```python
from build123d import *

# Parameters (mm, degrees)
BOSS_EXTRUDE1_DEPTH = 3
CUT_EXTRUDE1_REACH  = 69.03
SKETCH2_W           = 5
SKETCH2_H           = 35
BOSS_EXTRUDE8_DEPTH = 3
MIRROR1_DEPTH       = 3
FILLET1_R           = 2
FILLET2_R           = 10
FILLET3_R           = 6
FILLET4_R           = 1


# Read off the part's stored shape, not the designer's step: Mirror1
with BuildPart() as part:
    # Sketch1 → Boss-Extrude1 (new body)
    with BuildSketch(Plane.XY):
        with BuildLine():
            Line((-1.51, 0), (0, 0))
            Line((0, 0), (0, 5))
            Line((0, 5), (-1.51, 5))
            Line((-1.51, 5), (-1.51, 7))
            ThreePointArc((-1.51, 7), (-26.381774629, 5.897879108), (-50, -1.976082663))
            ThreePointArc((-50, -1.976082663), (-51.828078002, -17.5), (-50, -33.023917337))
            ThreePointArc((-50, -33.023917337), (-26.381774629, -40.897879108), (-1.51, -42))
            Line((-1.51, -42), (-1.51, -40))
            Line((-1.51, -40), (0, -40))
            Line((0, -40), (0, -35))
            Line((0, -35), (-1.51, -35))
            Line((-1.51, -35), (-1.51, -33))
            Line((-1.51, -33), (-1.51, -2))
            Line((-1.51, -2), (-1.51, 0))
        make_face()
    extrude(amount=BOSS_EXTRUDE1_DEPTH)

    # Sketch2 → Cut-Extrude1 (cut, up to next)
    with BuildSketch(Plane.XY.offset(3), mode=Mode.PRIVATE) as cut_extrude1_sk1:
        with BuildLine():
            ThreePointArc((-45.638636542, -5.430742036), (-46.828078002, -17.5), (-45.638636542, -29.569257964))
            ThreePointArc((-45.638636542, -29.569257964), (-26.536011476, -35.777357536), (-6.51, -37.329661985))
            Line((-6.51, -37.329661985), (-6.51, 2.329661985))
            ThreePointArc((-6.51, 2.329661985), (-26.536011476, 0.777357536), (-45.638636542, -5.430742036))
        make_face()
    cut_extrude1_tool1 = extrude(cut_extrude1_sk1.sketch, amount=-CUT_EXTRUDE1_REACH, mode=Mode.PRIVATE) & part.part
    # Sketch2 → Cut-Extrude1 (cut, up to next)
    with BuildSketch(Plane.XY.offset(3), mode=Mode.PRIVATE) as cut_extrude1_sk2:
        with Locations((-4.01, -17.5)):
            Rectangle(SKETCH2_W, SKETCH2_H)
    cut_extrude1_tool2 = extrude(cut_extrude1_sk2.sketch, amount=-CUT_EXTRUDE1_REACH, mode=Mode.PRIVATE) & part.part
    add(cut_extrude1_tool1.solids().sort_by_distance((-24.946194, -17.5, 3))[0], mode=Mode.SUBTRACT)
    add(cut_extrude1_tool2.solids().sort_by_distance((-4.01, -17.5, 3))[0], mode=Mode.SUBTRACT)

    # Sketch3 → Boss-Extrude8 (add)
    with BuildSketch(Plane.XY.offset(3)):
        with BuildLine():
            ThreePointArc((-32.612027687, -34.338487741), (-31.049231117, -34.753813219), (-29.478816537, -35.139334187))
            ThreePointArc((-29.478816537, -35.139334187), (-16.456843028, -24.361316901), (0, -20.5))
            Line((0, -20.5), (0, -14.5))
            ThreePointArc((0, -14.5), (-16.456843028, -10.638683099), (-29.478816537, 0.139334187))
            ThreePointArc((-29.478816537, 0.139334187), (-31.049231117, -0.246186781), (-32.612027687, -0.661512259))
            ThreePointArc((-32.612027687, -0.661512259), (-22.163998061, -10.798005795), (-8.780487851, -16.524390234))
            ThreePointArc((-8.780487851, -16.524390234), (-8, -17.499999784), (-8.780487429, -18.475609671))
            ThreePointArc((-8.780487429, -18.475609671), (-22.163997881, -24.201994085), (-32.612027687, -34.338487741))
        make_face()
    extrude(amount=-BOSS_EXTRUDE8_DEPTH)

    # Mirror1 outline → Mirror1 (add)
    with BuildSketch(Plane.XY):
        with BuildLine():
            ThreePointArc((29.478816537, -35.139334187), (18.069073524, -37.017473377), (6.51, -37.329661985))
            Line((6.51, -37.329661985), (6.51, -35))
            Line((6.51, -35), (0, -35))
            Line((0, -35), (0, -40))
            Line((0, -40), (1.51, -40))
            Line((1.51, -40), (1.51, -42))
            ThreePointArc((1.51, -42), (26.381774629, -40.897879108), (50, -33.023917337))
            ThreePointArc((50, -33.023917337), (51.828078002, -17.5), (50, -1.976082663))
            ThreePointArc((50, -1.976082663), (26.381774629, 5.897879108), (1.51, 7))
            Line((1.51, 7), (1.51, 5))
            Line((1.51, 5), (0, 5))
            Line((0, 5), (0, 0))
            Line((0, 0), (6.51, 0))
            Line((6.51, 0), (6.51, 2.329661985))
            ThreePointArc((6.51, 2.329661985), (18.069073524, 2.017473377), (29.478816537, 0.139334187))
            ThreePointArc((29.478816537, 0.139334187), (16.456843029, -10.638683099), (0, -14.5))
            Line((0, -14.5), (0, -20.5))
            ThreePointArc((0, -20.5), (16.456843029, -24.361316901), (29.478816537, -35.139334187))
        make_face()
        with BuildLine():
            ThreePointArc((45.638636542, -29.569257964), (39.22278835, -32.220063478), (32.612027687, -34.338487741))
            ThreePointArc((32.612027687, -34.338487741), (22.163998041, -24.201994192), (8.780487805, -18.475609756))
            ThreePointArc((8.780487805, -18.475609756), (8, -17.5), (8.780487805, -16.524390244))
            ThreePointArc((8.780487805, -16.524390244), (22.163998041, -10.798005808), (32.612027687, -0.661512259))
            ThreePointArc((32.612027687, -0.661512259), (39.22278835, -2.779936522), (45.638636542, -5.430742036))
            ThreePointArc((45.638636542, -5.430742036), (46.828078002, -17.5), (45.638636542, -29.569257964))
        make_face(mode=Mode.SUBTRACT)
    extrude(amount=MIRROR1_DEPTH)

    # Fillet1
    fillet1_edges = [part.edges().sort_by_distance(p)[0] for p in [
        (6.51, -35, 1.5),
        (6.51, 0, 1.5),
        (-6.51, 0, 1.5),
        (-6.51, -35, 1.5),
    ]]
    fillet(fillet1_edges, radius=FILLET1_R)

    # Fillet2
    fillet2_edges = [part.edges().sort_by_distance(p)[0] for p in [
        (-6.51, 2.329661985, 1.5),
        (6.51, 2.329661985, 1.5),
        (6.51, -37.329661985, 1.5),
        (-6.51, -37.329661985, 1.5),
    ]]
    fillet(fillet2_edges, radius=FILLET2_R)

    # Fillet3
    fillet3_edges = [part.edges().sort_by_distance(p)[0] for p in [
        (45.638636542, -5.430742036, 1.5),
        (45.638636542, -29.569257964, 1.5),
        (32.612027687, -0.661512259, 1.5),
        (32.612027687, -34.338487741, 1.5),
        (-50, -33.023917337, 1.5),
        (-50, -1.976082663, 1.5),
        (-45.638636542, -29.569257964, 1.5),
        (-45.638636542, -5.430742036, 1.5),
        (-32.612027687, -0.661512259, 1.5),
        (-32.612027687, -34.338487741, 1.5),
        (50, -1.976082663, 1.5),
        (50, -33.023917337, 1.5),
    ]]
    fillet(fillet3_edges, radius=FILLET3_R)

    # Fillet4
    fillet4_edges = [part.edges().sort_by_distance(p)[0] for p in [
        (29.478816537, 0.139334187, 1.5),
        (29.478816537, -35.139334187, 1.5),
        (-29.478816537, -35.139334187, 1.5),
        (-29.478816537, 0.139334187, 1.5),
    ]]
    fillet(fillet4_edges, radius=FILLET4_R)


solid = part.part
```
The model under review builds one solid part; all positions refer to its coordinate system, in mm. A direction names the side the tool comes from. Round coordinates to 2 decimals unless told otherwise and drop trailing zeros. Loops run counter-clockwise (first coordinate to the right, second up) from the corner with the lowest first, then second, coordinate; pieces in that order, holes last. Notation, with made-up numbers: (82.5, -36.5) - (101.5, -36.5) arc R18 cw to (101.5, -29.5) - close; hole circle Ø5 at (10, 7). An arc over 180 degrees is marked (long way). Use a Markdown table: item, result. Add a question column.
Q1. Add section B-B (y = -23). State the section outline as (x, z) points.
Q2. Add section D-D (y = 4). State the section outline as (x, z) points, plus the area to 3 significant figures.
Q3. The part is to be moulded in two halves that separate along X. For faces 5 (the face through (0, -19, 0)), 6 (the face through (51.828, -17.676, 1.479)), 7 (the face through (1.51, -41, 1)), say which applies: pulls with the +X half, pulls with the -X half, needs draft (parallel to the pull), parting line crosses it, or undercut.
Q4. Machinability: for faces 1 (the face through (-1.51, 6, 1)), 2 (the face through (-51.828, -17.324, 1.479)), 3 (the face through (39.68, -32.05, 1.48)), 4 (the face through (0, -40, 1)), which of the approach directions +Z, -Z, +X, -X, +Y, -Y give a long, thin tool a straight path to every point of the face, cutting with its end or side? Answer none if there is none.
Q5. Add section C-C (z = 0.8). State how many separate pieces and enclosed holes the cut face has, plus the area to 3 significant figures.
Q6. Insertion check: pin 1 Ø0.9 at (x, z) = (-0.5, 2) entering from +Y; pin 2 Ø1.5 at (x, z) = (0.5, 1.5) entering from -Y. Each pin has a flat end and moves straight along its axis. Give the tip position at first contact, or say it passes through.
Q7. For probe 1 along Y at (x, z) = (-1, 1.3); probe 2 along Y at (x, z) = (23, 0.5); probe 3 along Y at (x, z) = (21.5, 1.9), list the stretches that pass through material, from the lowest coordinate up.
Q8. Add section A-A (x = -21). State the section outline as (y, z) points, plus the area to 3 significant figures.
Worked answers:
| question | item | result |
|---|---|---|
| 1 | outline | (-51.6, 0) - (-46.58, 0) - (-46.58, 3) - (-51.6, 3) - close; (-20.24, 0) - (-13.37, 0) - (-13.37, 3) - (-20.24, 3) - close; (13.37, 0) - (20.24, 0) - (20.24, 3) - (13.37, 3) - close; (46.58, 0) - (51.6, 0) - (51.6, 3) - (46.58, 3) - close |
| 2 | outline | (-34.51, 0) - (34.51, 0) - (34.51, 3) - (-34.51, 3) - close |
| 2 | area | 207 mm² |
| 3 | face 5 | needs draft |
| 3 | face 6 | pulls with the +X half |
| 3 | face 7 | undercut |
| 4 | face 1 | +Z, -Z, +Y |
| 4 | face 2 | +Z, -Z, -X |
| 4 | face 3 | +Z, -Z |
| 4 | face 4 | +Z, -Z, -Y |
| 5 | separate pieces | 1 |
| 5 | enclosed holes | 4 |
| 5 | area | 1,770 mm² |
| 6 | pin 1 | y = 5 |
| 6 | pin 2 | y = -40 |
| 7 | probe 1 | -40 to -35, -20.51 to -14.49, 0 to 5 |
| 7 | probe 2 | -41.46 to -36.4, -28.52 to -24.77, -10.23 to -6.48, 1.4 to 6.46 |
| 7 | probe 3 | -41.66 to -36.62, -27.39 to -23.77, -11.23 to -7.61, 1.62 to 6.66 |
| 8 | outline | (-41.73, 0) - (-36.69, 0) - (-36.69, 3) - (-41.73, 3) - close; (-27.04, 0) - (-23.46, 0) - (-23.46, 3) - (-27.04, 3) - close; (-11.54, 0) - (-7.96, 0) - (-7.96, 3) - (-11.54, 3) - close; (1.69, 0) - (6.73, 0) - (6.73, 3) - (1.69, 3) - close |
| 8 | area | 51.7 mm² |
